Source: CAD feature listing. Evaluate the final solid. Frame: model axes, mm. Round coordinates to 2 decimals unless told otherwise and drop trailing zeros. Order: outer loops, then holes, each group sorted by start corner. A loop starts at its lowest first (then second) coordinate and runs counter-clockwise, first axis right, second up. Notation, with made-up numbers: (73, 25) -> (95, 25) arc R16 cw to (95, 35) -> close; hole circle Ø8 at (66.5, -26.75). An arc over 180 degrees is marked (long way). Write item = value, one per line. Start each with the question number.
(1) Cut plane A-A on x = 0. Return the cut outline in (y, z).
(2) Ray query, line 1 (Y direction, x = 0, z = 2.4); line 2 (Y direction, x = 0, z = 1.65); line 3 (X direction, y = 1, z = 0.55). Return the intervals inside material, ascending.
(3) Cut plane B-B on y = -163.5. Return the cut outline in (x, z).
(4) Contact query for flat-ended pins moving along their axis: pin 1 Ø2 at (y, z) = (-177.5, 2.5) entering from -X; pin 2 Ø4 at (x, y) = (-4, -36.5) entering from +Z; pin 3 Ø3 at (y, z) = (-167.5, 3.5) entering from -X; pin 4 Ø1.1 at (y, z) = (-10.5, 4) entering from +X. Output: stop coordinate, or through.
(5) Cut plane D-D on x = 61. Return the cut outline in (y, z).
(6) Cut plane C-C on z = 2.8. Give the number of separate pieces and of enclosed holes in the cut face, then the cut area to 3 significant figures.
from build123d import *

# Parameters (mm, degrees)
BOSS_EXTRUDE1_DEPTH = 5.588
CUT_EXTRUDE1_DEPTH  = 260.036579176
CUT_EXTRUDE2_DEPTH  = 260.036579176
CUT_EXTRUDE3_DEPTH  = 260.036579176
CAVITY1_START       = 1.9558
CAVITY1_OUTLINE_W   = 15.946260678
CAVITY1_OUTLINE_H   = 5.08
CAVITY1_OUTLINE_W_2 = 5.08
CAVITY1_OUTLINE_H_2 = 14.202900977
CAVITY1_OUTLINE_H_3 = 13.341513611
CAVITY1_DEPTH       = 3.6322
CAVITY2_OUTLINE_R   = 10.875645
CAVITY2_DEPTH       = 5.588


# Read off the part's stored shape, not the designer's step: Cavity1, Cavity2
with BuildPart() as part:
    # Sketch1 → Boss-Extrude1 (new body)
    with BuildSketch(Plane.XY):
        with BuildLine():
            Line((65.678975516, 61.334336478), (-65.678975516, 61.334336478))
            ThreePointArc((-65.678975516, 61.334336478), (-75.399134698, 59.400876604), (-83.639487758, 53.89484872))
            Line((-83.639487758, 53.89484872), (-132.260512242, 5.273824236))
            ThreePointArc((-132.260512242, 5.273824236), (-137.766540126, -2.966528824), (-139.7, -12.686688006))
            Line((-139.7, -12.686688006), (-139.7, -114.753454114))
            ThreePointArc((-139.7, -114.753454114), (-137.766540126, -124.473613296), (-132.260512242, -132.713966356))
            Line((-132.260512242, -132.713966356), (-54.348302834, -210.626175764))
            ThreePointArc((-54.348302834, -210.626175764), (-46.107949774, -216.132203648), (-36.387790592, -218.065663522))
            Line((-36.387790592, -218.065663522), (36.387790592, -218.065663522))
            ThreePointArc((36.387790592, -218.065663522), (46.107949774, -216.132203648), (54.348302834, -210.626175764))
            Line((54.348302834, -210.626175764), (132.260512242, -132.713966356))
            ThreePointArc((132.260512242, -132.713966356), (137.766540126, -124.473613296), (139.7, -114.753454114))
            Line((139.7, -114.753454114), (139.7, -12.686688006))
            ThreePointArc((139.7, -12.686688006), (137.766540126, -2.966528824), (132.260512242, 5.273824236))
            Line((132.260512242, 5.273824236), (83.639487758, 53.89484872))
            ThreePointArc((83.639487758, 53.89484872), (75.399134698, 59.400876604), (65.678975516, 61.334336478))
        make_face()
    extrude(amount=BOSS_EXTRUDE1_DEPTH)

    # Sketch3 → Cut-Extrude1 (cut, through all)
    with BuildSketch(Plane(origin=(0, 0, 0), x_dir=(-1, 0, 0), z_dir=(0, 0, -1))):
        with BuildLine():
            Line((-17.5895, 16.256), (-17.5895, 23.876))
            ThreePointArc((-17.5895, 23.876), (-16.1925, 25.273), (-14.7955, 23.876))
            Line((-14.7955, 23.876), (-14.7955, 16.256))
            ThreePointArc((-14.7955, 16.256), (-16.1925, 14.859), (-17.5895, 16.256))
        make_face()
        with BuildLine():
            Line((14.7955, 16.256), (14.7955, 23.876))
            ThreePointArc((14.7955, 23.876), (16.1925, 25.273), (17.5895, 23.876))
            Line((17.5895, 23.876), (17.5895, 16.256))
            ThreePointArc((17.5895, 16.256), (16.1925, 14.859), (14.7955, 16.256))
        make_face()
        with BuildLine():
            Line((-17.5895, -16.256), (-17.5895, -8.636))
            ThreePointArc((-17.5895, -8.636), (-16.1925, -7.239), (-14.7955, -8.636))
            Line((-14.7955, -8.636), (-14.7955, -16.256))
            ThreePointArc((-14.7955, -16.256), (-16.1925, -17.653), (-17.5895, -16.256))
        make_face()
    extrude(amount=-CUT_EXTRUDE1_DEPTH, mode=Mode.SUBTRACT)

    # Sketch6 → Cut-Extrude2 (cut, through all)
    with BuildSketch(Plane(origin=(0, 0, 0), x_dir=(-1, 0, 0), z_dir=(0, 0, -1))):
        with BuildLine():
            Line((-11.1125, 0), (-11.1125, 7.62))
            ThreePointArc((-11.1125, 7.62), (0, 18.7325), (11.1125, 7.62))
            Line((11.1125, 7.62), (11.1125, 0))
            ThreePointArc((11.1125, 0), (0, -11.1125), (-11.1125, 0))
        make_face()
    extrude(amount=-CUT_EXTRUDE2_DEPTH, mode=Mode.SUBTRACT)

    # Sketch5 → Cut-Extrude3 (cut, through all)
    with BuildSketch(Plane(origin=(0, 0, 0), x_dir=(-1, 0, 0), z_dir=(0, 0, -1))):
        with BuildLine():
            Line((14.7955, -16.256), (14.7955, -8.636))
            ThreePointArc((14.7955, -8.636), (16.1925, -7.239), (17.5895, -8.636))
            Line((17.5895, -8.636), (17.5895, -16.256))
            ThreePointArc((17.5895, -16.256), (16.1925, -17.653), (14.7955, -16.256))
        make_face()
    extrude(amount=-CUT_EXTRUDE3_DEPTH, mode=Mode.SUBTRACT)

    # Cavity1 outline → Cavity1 (cut)
    with BuildSketch(Plane.XY.offset(CAVITY1_START)):
        with Locations((-0.487430597, 35.56)):
            Rectangle(CAVITY1_OUTLINE_W, CAVITY1_OUTLINE_H)
        with Locations((-0.487430597, -35.56)):
            Rectangle(CAVITY1_OUTLINE_W, CAVITY1_OUTLINE_H)
        with Locations((29.21, 13.086687708)):
            Rectangle(CAVITY1_OUTLINE_W_2, CAVITY1_OUTLINE_H_2)
        with Locations((-29.21, 13.517381391)):
            Rectangle(CAVITY1_OUTLINE_W_2, CAVITY1_OUTLINE_H_3)
        with Locations((29.21, -13.517381391)):
            Rectangle(CAVITY1_OUTLINE_W_2, CAVITY1_OUTLINE_H_3)
        with Locations((-29.21, -13.086687708)):
            Rectangle(CAVITY1_OUTLINE_W_2, CAVITY1_OUTLINE_H_2)
    extrude(amount=CAVITY1_DEPTH, mode=Mode.SUBTRACT)

    # Cavity2 outline → Cavity2 (cut)
    with BuildSketch(Plane.XY):
        with Locations((0, -78.365663522)):
            Circle(CAVITY2_OUTLINE_R)
    extrude(amount=CAVITY2_DEPTH, mode=Mode.SUBTRACT)


solid = part.part
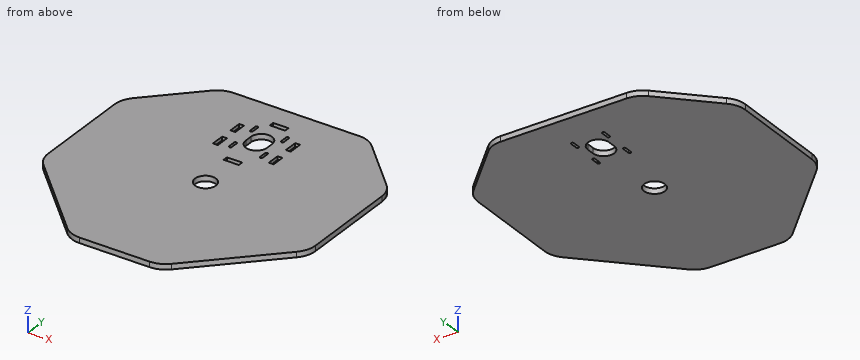
Evaluation:
q1.outline = (-218.07, 0) -> (-89.24, 0) -> (-89.24, 5.59) -> (-218.07, 5.59) -> close; (-67.49, 0) -> (-11.11, 0) -> (-11.11, 5.59) -> (-33.02, 5.59) -> (-33.02, 1.96) -> (-38.1, 1.96) -> (-38.1, 5.59) -> (-67.49, 5.59) -> close; (18.73, 0) -> (61.33, 0) -> (61.33, 5.59) -> (38.1, 5.59) -> (38.1, 1.96) -> (33.02, 1.96) -> (33.02, 5.59) -> (18.73, 5.59) -> close
q2.line_1 = -218.07 to -89.24, -67.49 to -38.1, -33.02 to -11.11, 18.73 to 33.02, 38.1 to 61.33
q2.line_2 = -218.07 to -89.24, -67.49 to -11.11, 18.73 to 61.33
q2.line_3 = -135.7 to -11.11, 11.11 to 135.7
q3.outline = (-101.47, 0) -> (101.47, 0) -> (101.47, 5.59) -> (-101.47, 5.59) -> close
q4.pin_1 = -88.47
q4.pin_2 = 5.59
q4.pin_3 = -98.97
q4.pin_4 = 139.65
q5.outline = (-203.97, 0) -> (61.33, 0) -> (61.33, 5.59) -> (-203.97, 5.59) -> close
q6.separate_pieces = 1
q6.enclosed_holes = 12
q6.area = 63,800 mm^2
